```python
from build123d import *

# Parameters (mm, degrees)
SKETCH1_R           = 65
BOSS_EXTRUDE1_DEPTH = 3
SKETCH2_R           = 3
CUT_EXTRUDE1_DEPTH  = 4
CIRPATTERN1_COUNT   = 4


with BuildPart() as part:
    # Sketch1 → Boss-Extrude1 (new body)
    with BuildSketch(Plane(origin=(0, 0, 0), x_dir=(1, 0, 0), z_dir=(0, 1, 0))):
        Circle(SKETCH1_R)
    extrude(amount=BOSS_EXTRUDE1_DEPTH)

    # Sketch2 → Cut-Extrude1 (cut, through all)
    with BuildSketch(Plane(origin=(0, 3, 0), x_dir=(1, 0, 0), z_dir=(0, 1, 0))):
        with Locations((0, 55)):
            Circle(SKETCH2_R)
    cut_extrude1 = extrude(amount=-CUT_EXTRUDE1_DEPTH, mode=Mode.SUBTRACT)

    # CirPattern1: Cut-Extrude1 ×4 about axis
    cirpattern1_axis = Axis((0, 0, 0), (0, 1, 0))
    for i in range(1, CIRPATTERN1_COUNT):
        add(cut_extrude1.rotate(cirpattern1_axis, i * 360 / CIRPATTERN1_COUNT), mode=Mode.SUBTRACT)


solid = part.part
```
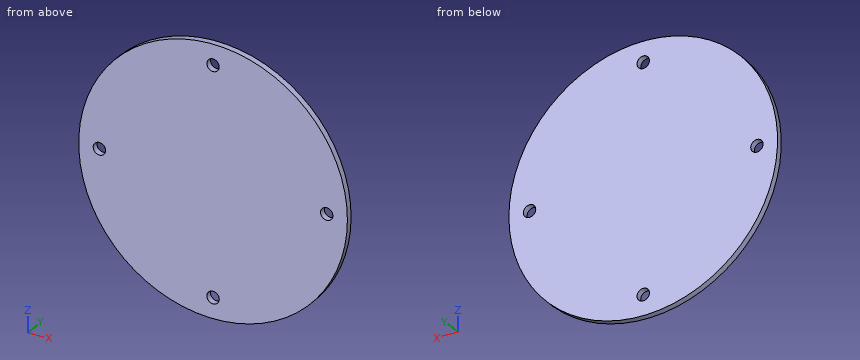
Work out the finished part from the listing and answer in its coordinate system (mm). Round coordinates to 2 decimals unless told otherwise and drop trailing zeros. Loops run counter-clockwise (first coordinate to the right, second up) from the corner with the lowest first, then second, coordinate; pieces in that order, holes last.
(1) The part is cut by section D-D, the plane y = 0.6. Give the vertices of the cut face in (x, z), and give its area (3 significant figures).
Computed values:
outline: circle Ø130 at (0, 0); hole circle Ø6 at (-55, 0); hole circle Ø6 at (0, -55); hole circle Ø6 at (0, 55); hole circle Ø6 at (55, 0)
area: 13,200 mm2
(2) Find the intervals of material crossed by L1, parallel to X at y = 1.1, z = 0; L2, parallel to X at y = 0.2, z = -2, in increasing order.
Computed values:
L1: x = -65 to -58, -52 to 52, 58 to 65
L2: x = -64.97 to -57.24, -52.76 to 52.76, 57.24 to 64.97
(3) The part is cut by section A-A, the plane z = 0. Give the vertices of the cut face in (x, y).
Computed values:
outline: (-65, 0) - (-58, 0) - (-58, 3) - (-65, 3) - close; (-52, 0) - (52, 0) - (52, 3) - (-52, 3) - close; (58, 0) - (65, 0) - (65, 3) - (58, 3) - close
(4) The part is cut by section B-B, the plane x = 0. Give the vertices of the cut face in (y, z).
Computed values:
outline: (0, -65) - (3, -65) - (3, -58) - (0, -58) - close; (0, -52) - (3, -52) - (3, 52) - (0, 52) - close; (0, 58) - (3, 58) - (3, 65) - (0, 65) - close
(5) Each of these flat-tipped pins is pushed along its axis until it touches: P1, Ø1.5, axis at x = 11.5, y = 0.5, coming from the +Z side; P2, Ø1, axis at x = 34, y = 1, coming from the +Z side; P3, Ø1.5, axis at x = 18, y = 0.5, coming from the +Z side. Where does it stop, or does it pass through?
Computed values:
P1: stops at z = 64.1
P2: stops at z = 55.7
P3: stops at z = 62.67
(6) The part is cut by section C-C, the plane z = -55. Give the vertices of the cut face in (x, y), and give its area (3 significant figures).
Computed values:
outline: (-34.64, 0) - (-3, 0) - (-3, 3) - (-34.64, 3) - close; (3, 0) - (34.64, 0) - (34.64, 3) - (3, 3) - close
area: 190 mm2
